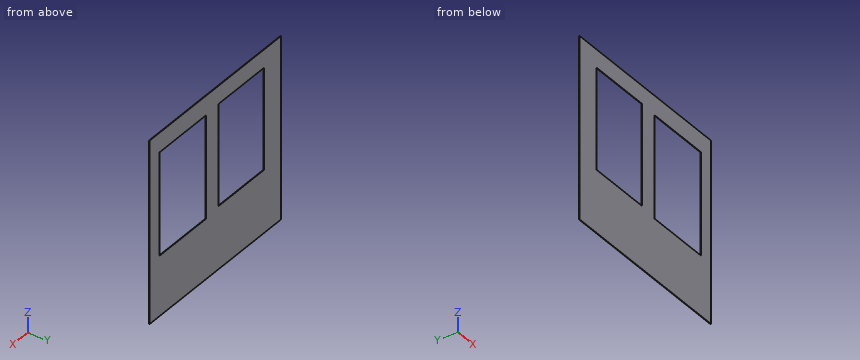
```python
from build123d import *

# Parameters (mm, degrees)
F0_W     = 114.3
F0_H     = 114.3
F1_DEPTH = 0.3
F2_W     = 39.628732
F2_H     = 63.614545
F3_DEPTH = 0.301
F4_W     = 40.832126
F4_H     = 64.454022
F5_DEPTH = 0.301


with BuildPart() as f1:
    # F0 (on Front) → F1 (new body)
    with BuildSketch(Plane.XZ):
        with Locations((6.831163, 6.801479)):
            Rectangle(F0_W, F0_H)
    extrude(amount=F1_DEPTH)

    # F2 (on face) → F3 (cut, through all)
    with BuildSketch(Plane.XZ.offset(0.3)):
        with Locations((-15.981431, 20.791628)):
            Rectangle(F2_W, F2_H)
    extrude(amount=-F3_DEPTH, mode=Mode.SUBTRACT)

    # F4 (on face) → F5 (cut, through all)
    with BuildSketch(Plane.XZ.offset(0.3)):
        with Locations((35.110194, 19.508778)):
            Rectangle(F4_W, F4_H)
    extrude(amount=-F5_DEPTH, mode=Mode.SUBTRACT)


solid = f1.part
```
Model file for the job. Use its own axes, mm. Coordinates: 2 decimals unless noted, no trailing zeros. Write each loop counter-clockwise with the first axis right and the second up, starting at its lowest first coordinate (ties: lowest second). Pieces come first, ordered by that corner, then holes. Notation, with made-up numbers: (78, 26) - (128, 26) arc R34 cw to (128, 58) - close; hole circle Ø4 at (21, 67). An arc over 180 degrees is marked (long way). One line per question, with ' | ' between items. Start each with the question number.
Q1. Cut at A-A, the plane x = 36.5. List the corners of the cut face in (y, z), then the cut area to 3 significant figures.
Q2. Cut at D-D, the plane x = -16. List the corners of the cut face in (y, z), then the cut area to 3 significant figures.
Q3. Drill centre lines: line 1 (X direction, y = -0.2, z = 7); line 2 (Z direction, x = -18, y = -0.05); line 3 (Z direction, x = 45, y = -0.2). Where is each one in solid material? Low to high. Write a range as [from, to].
Q4. Cut at B-B, the plane z = -2.5. List the corners of the cut face in (x, y), then the cut area to 3 significant figures.
Q5. Cut at C-C, the plane y = -0.2. List the corners of the cut face in (x, z), then the cut area to 3 significant figures.
Answer below:
1) outline: (-0.3, -50.35) - (0, -50.35) - (0, -12.72) - (-0.3, -12.72) - close; (-0.3, 51.74) - (0, 51.74) - (0, 63.95) - (-0.3, 63.95) - close | area: 15.0 mm^2
2) outline: (-0.3, -50.35) - (0, -50.35) - (0, -11.02) - (-0.3, -11.02) - close; (-0.3, 52.6) - (0, 52.6) - (0, 63.95) - (-0.3, 63.95) - close | area: 15.2 mm^2
3) line 1: [-50.32, -35.8], [3.83, 14.69], [55.53, 63.98] | line 2: [-50.35, -11.02], [52.6, 63.95] | line 3: [-50.35, -12.72], [51.74, 63.95]
4) outline: (-50.32, -0.3) - (-35.8, -0.3) - (-35.8, 0) - (-50.32, 0) - close; (3.83, -0.3) - (14.69, -0.3) - (14.69, 0) - (3.83, 0) - close; (55.53, -0.3) - (63.98, -0.3) - (63.98, 0) - (55.53, 0) - close | area: 10.2 mm^2
5) outline: (-50.32, -50.35) - (63.98, -50.35) - (63.98, 63.95) - (-50.32, 63.95) - close; hole (-35.8, -11.02) - (3.83, -11.02) - (3.83, 52.6) - (-35.8, 52.6) - close; hole (14.69, -12.72) - (55.53, -12.72) - (55.53, 51.74) - (14.69, 51.74) - close | area: 7,910 mm^2
